Input: dimensioned drawing with shaded views. Units: mm. Origin: part minimum x, y, z. A direction names the side the tool comes from. Give positions to 0.01 mm unless a question says otherwise; leave off trailing zeros. Loops run counter-clockwise (first coordinate to the right, second up) from the corner with the lowest first, then second, coordinate; pieces in that order, holes last. Notation, with made-up numbers: (22, 17) -> (29, 17) arc R21 cw to (29, 36) -> close; hole circle Ø5 at (43, 39.5). An arc over 180 degrees is marked (long way). Answer in a Markdown table with one row per item. Add a question column.
1) Section query C-C (x = 313). Return the cut outline in (y, z).
2) Section query A-A (x = 250). Return the cut outline in (y, z).
3) First-contact query: P1, Ø6, axis at x = 314.5, z = 330, coming from the -Y side; P2, Ø4, axis at y = 264, z = 239, coming from the +X side. Flat tips, straight axial feed; report the tip coordinate or a pass-through.
4) Section query B-B (y = 250). Return the cut outline in (x, z), plus the area to 3 significant figures.
5) Draft query along Z for the marked faces 6, 7, 8 and 9. Return one class per face: +Z half, -Z half, draft (parallel to the pull), parting line (faces both ways), or undercut.
6) Section query D-D (z = 418). Return the cut outline in (x, y).
7) Access query for the marked faces 1, 2, 3, 4 and 5. Directions: +Z, -Z, +X, -X, +Y, -Y. A direction counts if a zero-diameter tool reaches every point of the face in a straight line with its end or side. Return the directions, or none.
8) Line query: line 1 (Z direction, x = 250, y = 334); line 2 (Y direction, x = 317, z = 440); line 3 (Z direction, x = 438, y = 96.5). Output: solid intervals per line, ascending. Write a range as from..to.
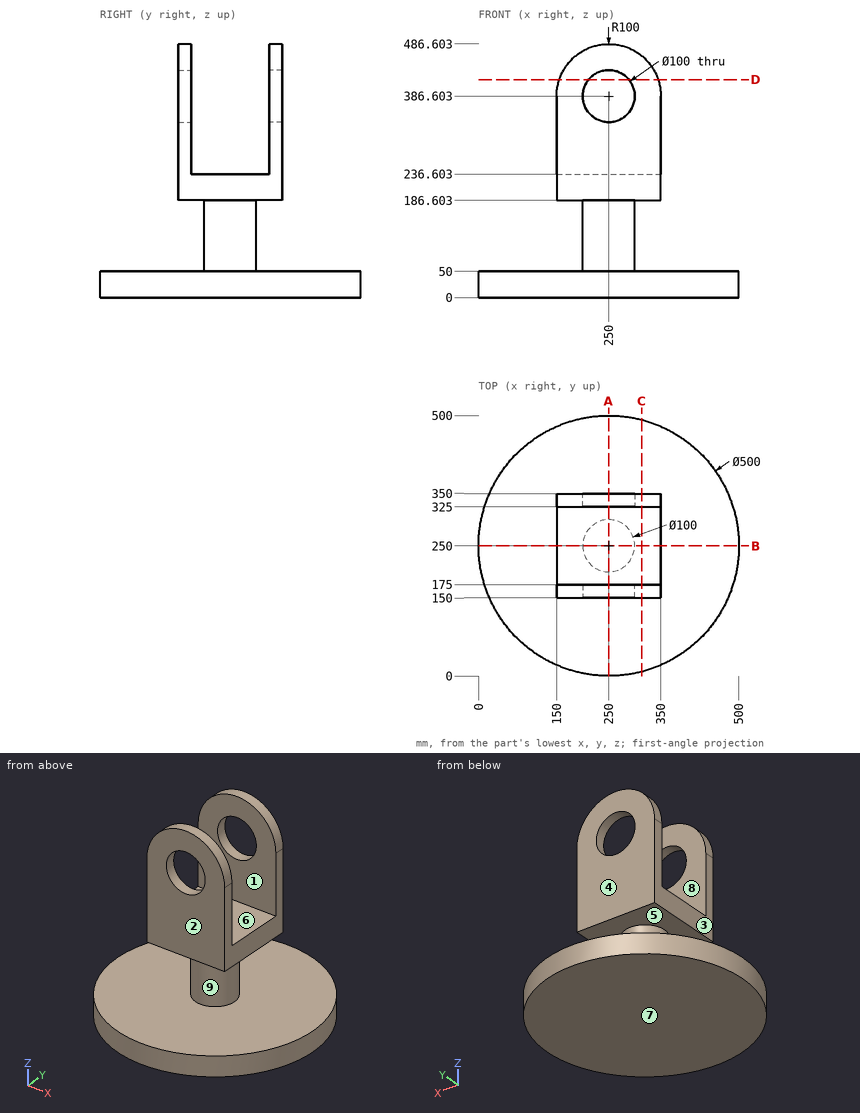
Evaluation:
| question | item | result |
|---|---|---|
| 1 | outline | (8.07, 0) -> (491.93, 0) -> (491.93, 50) -> (8.07, 50) -> close; (150, 186.6) -> (350, 186.6) -> (350, 464.26) -> (325, 464.26) -> (325, 236.6) -> (175, 236.6) -> (175, 464.26) -> (150, 464.26) -> close |
| 2 | outline | (0, 0) -> (500, 0) -> (500, 50) -> (300, 50) -> (300, 186.6) -> (350, 186.6) -> (350, 336.6) -> (325, 336.6) -> (325, 236.6) -> (175, 236.6) -> (175, 336.6) -> (150, 336.6) -> (150, 186.6) -> (200, 186.6) -> (200, 50) -> (0, 50) -> close; (150, 436.6) -> (175, 436.6) -> (175, 486.6) -> (150, 486.6) -> close; (325, 436.6) -> (350, 436.6) -> (350, 486.6) -> (325, 486.6) -> close |
| 3 | P1 | y = 150 |
| 3 | P2 | through |
| 4 | outline | (0, 0) -> (500, 0) -> (500, 50) -> (300, 50) -> (300, 186.6) -> (350, 186.6) -> (350, 236.6) -> (150, 236.6) -> (150, 186.6) -> (200, 186.6) -> (200, 50) -> (0, 50) -> close |
| 4 | area | 48,700 mm² |
| 5 | face 6 | +Z half |
| 5 | face 7 | -Z half |
| 5 | face 8 | draft |
| 5 | face 9 | undercut |
| 6 | outline | (155.06, 150) -> (211.09, 150) -> (211.09, 175) -> (155.06, 175) -> close; (155.06, 325) -> (211.09, 325) -> (211.09, 350) -> (155.06, 350) -> close; (288.91, 150) -> (344.94, 150) -> (344.94, 175) -> (288.91, 175) -> close; (288.91, 325) -> (344.94, 325) -> (344.94, 350) -> (288.91, 350) -> close |
| 7 | face 1 | +Z, +X, -X |
| 7 | face 2 | +Z, +X, -X, -Y |
| 7 | face 3 | +Z, -X, +Y, -Y |
| 7 | face 4 | +Z, +X, -X, +Y |
| 7 | face 5 | none |
| 8 | line 1 | 0..50, 186.6..336.6, 436.6..486.6 |
| 8 | line 2 | 150..175, 325..350 |
| 8 | line 3 | 0..50 |
